Input: part model. Units: mm. Frame: model coordinates. A direction names the side the tool comes from. Round coordinates to 2 decimals unless told otherwise and drop trailing zeros. Loops run counter-clockwise (first coordinate to the right, second up) from the corner with the lowest first, then second, coordinate; pieces in that order, holes last. Notation, with made-up numbers: (-13, 32.5) -> (45, 32.5) arc R24 ccw to (45, 62.5) -> close; hole circle Ø3 at (61.25, -27). An arc over 180 degrees is marked (long way). Answer in a Markdown table with one row per item. Add a question column.
Q1. Ray query, L1, parallel to Y at x = 6.55, z = 9; L2, parallel to Z at x = 7, y = 0.5; L3, parallel to X at y = 5.5, z = 8.75. Return the intervals inside material, ascending. Write a range as from..to.
Q2. Section C-C, the plane x = 6.25. Output: boundary loops of the cut face in (y, z).
Q3. Section A-A, the plane z = 9. Output: boundary loops of the cut face in (x, y), and give its area (3 significant figures).
Q4. Section D-D, the plane z = 12.75. Output: boundary loops of the cut face in (x, y).
Q5. Reachability of faces 5 (the face through (0.269, 0.154, -8.924)), 6 (the face through (0, 6, -11.428)), 7 (the face through (2, 11, -9)), 8 (the face through (0, 0, -9.428)), 9 (the face through (-5.5, 0, 12)) from +Z, -Z, +X, -X, +Y, -Y: full face, straight path, thin tool, end or side. Return the list, or none.
Q6. Mould query, pull axis Z, two halves, no side actions, for faces 1 (the face through (0, 1.4, -10)), 2 (the face through (2.5, 6, -12)), 3 (the face through (-8, 0, 15)), 4 (the face through (0, -6, -11.428)). Classes: pulls with the +Z half, pulls with the -Z half, needs draft (parallel to the pull), parting line crosses it, or undercut.
Q7. Section B-B, the plane y = 0. Output: boundary loops of the cut face in (x, z).
Q8. Pin query (flat end, axial travel): pin 1 (4.5 mm diameter, centred on y = 0, z = 9, fed in from +X). Return the tip coordinate at first contact, or that it passes through.
```python
from build123d import *

# Parameters (mm, degrees)
BOSS_EXTRUDE1_DEPTH = 11
CUT_EXTRUDE1_REACH  = 30.128
SKETCH2_R           = 2.55
SKETCH4_W           = 2
SKETCH4_H           = 2.8
CUT_EXTRUDE3_DEPTH  = 21.1
SKETCH5_W           = 5
SKETCH5_H           = 5
CUT_EXTRUDE5_DEPTH  = 2


with BuildPart() as part:
    # Sketch1 → Boss-Extrude1 (new, symmetric)
    with BuildSketch(Plane(origin=(0, 0, 0), x_dir=(1, 0, 0), z_dir=(0, 1, 0))):
        with BuildLine():
            Line((-5.5, -15), (-10.55, -15))
            Line((-10.55, -15), (-10.55, 13.42813746))
            Line((-10.55, 13.42813746), (10.55, 13.42813746))
            Line((10.55, 13.42813746), (10.55, -15))
            Line((10.55, -15), (5.5, -15))
            Line((5.5, -15), (5.5, -5))
            ThreePointArc((5.5, -5), (0, 8.92813746), (-5.5, -5))
            Line((-5.5, -5), (-5.5, -15))
        make_face()
    extrude(amount=BOSS_EXTRUDE1_DEPTH, both=True)

    # Cut-Extrude1: up to this face of the body (flat: up to its plane)
    cut_extrude1_end = Plane(part.part.faces().sort_by_distance((-10.55, 0, 0.78593127))[0])
    # Sketch2 → Cut-Extrude1 (cut, up to the picked face)
    with BuildSketch(Plane(origin=(10.55, 0, 0), x_dir=(0, 0, -1), z_dir=(1, 0, 0)), mode=Mode.PRIVATE) as cut_extrude1_sk1:
        with Locations((-9, 0)):
            Circle(SKETCH2_R)
    cut_extrude1_tool1 = split(extrude(cut_extrude1_sk1.sketch, amount=-CUT_EXTRUDE1_REACH, mode=Mode.PRIVATE), bisect_by=cut_extrude1_end, keep=Keep.BOTH, mode=Mode.PRIVATE)
    add(cut_extrude1_tool1.solids().sort_by(Axis((10.55, 0, 9), (-1, 0, 0)))[0], mode=Mode.SUBTRACT)

    # Sketch4 → Cut-Extrude3 (cut)
    with BuildSketch(Plane(origin=(10.55, 0, 0), x_dir=(0, 0, -1), z_dir=(1, 0, 0))):
        with Locations((10.42813746, 0)):
            Rectangle(SKETCH4_W, SKETCH4_H)
    extrude(amount=-CUT_EXTRUDE3_DEPTH, mode=Mode.SUBTRACT)

    # Sketch5 → Cut-Extrude5 (cut)
    with BuildSketch(Plane(origin=(0, 0, -13.42813746), x_dir=(-1, 0, 0), z_dir=(0, 0, -1))):
        with Locations((0, 6)):
            Rectangle(SKETCH5_W, SKETCH5_H)
        with Locations((0, -6)):
            Rectangle(SKETCH5_W, SKETCH5_H)
    extrude(amount=-CUT_EXTRUDE5_DEPTH, mode=Mode.SUBTRACT)


solid = part.part
```
Answer block:
| question | item | result |
|---|---|---|
| 1 | L1 | -11..-2.55, 2.55..11 |
| 1 | L2 | -13.43..-11.43, -9.43..-4.85, 3.1..6.5, 11.5..15 |
| 1 | L3 | -10.55..-5.5, 5.5..10.55 |
| 2 | outline | (-11, -13.43) -> (11, -13.43) -> (11, -5.95) -> (-11, -5.95) -> close; (-11, 4.2) -> (11, 4.2) -> (11, 15) -> (-11, 15) -> close; hole circle Ø5.1 at (0, 9); hole (-1.4, -11.43) -> (1.4, -11.43) -> (1.4, -9.43) -> (-1.4, -9.43) -> close |
| 3 | outline | (-10.55, -11) -> (-5.5, -11) -> (-5.5, -2.55) -> (-10.55, -2.55) -> close; (-10.55, 2.55) -> (-5.5, 2.55) -> (-5.5, 11) -> (-10.55, 11) -> close; (5.5, -11) -> (10.55, -11) -> (10.55, -2.55) -> (5.5, -2.55) -> close; (5.5, 2.55) -> (10.55, 2.55) -> (10.55, 11) -> (5.5, 11) -> close |
| 3 | area | 171 mm^2 |
| 4 | outline | (-10.55, -11) -> (-5.5, -11) -> (-5.5, 11) -> (-10.55, 11) -> close; (5.5, -11) -> (10.55, -11) -> (10.55, 11) -> (5.5, 11) -> close |
| 5 | face 5 | +Y, -Y |
| 5 | face 6 | -Z |
| 5 | face 7 | +Z, -Z, +X, -X, +Y |
| 5 | face 8 | +X, -X |
| 5 | face 9 | +Z, +Y, -Y |
| 6 | face 1 | undercut |
| 6 | face 2 | needs draft |
| 6 | face 3 | pulls with the +Z half |
| 6 | face 4 | pulls with the -Z half |
| 7 | outline | (-10.55, -13.43) -> (10.55, -13.43) -> (10.55, -11.43) -> (-10.55, -11.43) -> close; (-10.55, -9.43) -> (10.55, -9.43) -> (10.55, 6.45) -> (5.5, 6.45) -> (5.5, 5) arc R8.05 cw (long way) to (-5.5, 5) -> (-5.5, 6.45) -> (-10.55, 6.45) -> close; (-10.55, 11.55) -> (-5.5, 11.55) -> (-5.5, 15) -> (-10.55, 15) -> close; (5.5, 11.55) -> (10.55, 11.55) -> (10.55, 15) -> (5.5, 15) -> close |
| 8 | pin 1 | through |
